from build123d import *

# Parameters (mm, degrees)
F0_W     = 152.4
F0_H     = 133.35
F1_DEPTH = 3.175
F3_DEPTH = 3.175


with BuildPart() as f1:
    # F0 (on Top) → F1 (new body)
    with BuildSketch(Plane.XY):
        Rectangle(F0_W, F0_H)
    extrude(amount=F1_DEPTH)

    # F2 (on face) → F3 (join)
    with BuildSketch(Plane.XY.offset(3.175)):
        Polygon((-241.3, 292.1), (-241.3, 66.675), (-76.2, 66.675), (76.2, 66.675), (241.3, 66.675), (241.3, 292.1), align=None)
        Polygon((76.2, -66.675), (-76.2, -66.675), (-241.3, -66.675), (-241.3, -285.75), (241.3, -285.75), (241.3, -66.675), align=None)
    extrude(amount=-F3_DEPTH)


with BuildPart() as f4_1:
    # F4: copy of F1
    add(f1.part)


solid = f1.part
Verification items for the finished model (mm, model axes). Coordinates: 2 decimals unless noted, no trailing zeros. Write each loop counter-clockwise with the first axis right and the second up, starting at its lowest first coordinate (ties: lowest second). Pieces come first, ordered by that corner, then holes. Notation, with made-up numbers: (-32, 76) - (19, 76) arc R21 cw to (19, 107) - close; hole circle Ø3 at (16, 72.25). An arc over 180 degrees is marked (long way). Answer as a JSON object with one key per item and string values.
(1) Thickness scan on line 1 along Y through (x, z) = (-100, 3) (3 decimals); line 2 along X through (y, z) = (-22.5, 2.5). Record the ranges inside material, lowest first.
Report:
{"line 1": "-285.75 to -66.675, 66.675 to 292.1", "line 2": "-76.2 to 76.2"}
(2) Cross-section at A-A on x = -114. Record the cut outline in (y, z) (3 decimals).
Report:
{"outline": "(-285.75, 0) - (-66.675, 0) - (-66.675, 3.175) - (-285.75, 3.175) - close; (66.675, 0) - (292.1, 0) - (292.1, 3.175) - (66.675, 3.175) - close"}
(3) Cross-section at B-B on z = 1.8. Record the cut outline in (x, y) (3 decimals), plus the area to 3 significant figures.
Report:
{"outline": "(-241.3, -285.75) - (241.3, -285.75) - (241.3, -66.675) - (76.2, -66.675) - (76.2, 66.675) - (241.3, 66.675) - (241.3, 292.1) - (-241.3, 292.1) - (-241.3, 66.675) - (-76.2, 66.675) - (-76.2, -66.675) - (-241.3, -66.675) - close", "area": "235,000 mm^2"}
